Autodesk Inventor part; units mm, degrees
ref_plane "YZ Plane" through (0, 0, 0) normal (1, 0, 0) x (0, 1, 0)
ref_plane "XZ Plane" through (0, 0, 0) normal (0, 1, 0) x (-1, 0, 0)
ref_plane "XY Plane" through (0, 0, 0) normal (0, 0, 1) x (1, 0, 0)
sketch "Sketch1" plane through (0, 0, 0) normal (0, 0, 1) x (1, 0, 0)
  line L0 (-85, 15) -> (85, 15)
  line L1 (85, 15) -> (85, -15)
  line L2 (85, -15) -> (-85, -15)
  line L3 (-85, -15) -> (-85, 15)
  point P0 (0, 0)
  dimension "d0" = 30
  dimension "d1" = 170
  dimension "d2" = 85
  dimension "d3" = 15
extrude "Extrusion1" add sketch "Sketch1" along normal blind 10
sketch "Sketch2" plane through (0, 0, 10) normal (0, 0, 1) x (1, 0, 0)
  point P0 (0, 0)
  point P1 (-37.5, 0)
  point P2 (-12.5, 0)
  point P3 (12.5, 0)
  point P4 (37.5, 0)
  dimension "d30" = 25
  dimension "d31" = 25
  dimension "d32" = 25
  dimension "d33" = 12.5
hole "Hole1" at (-37.5, 0, 10) at (-12.5, 0, 10) at (12.5, 0, 10) at (37.5, 0, 10) direction (0, 0, -1) diameter 6.6 end through all counterbore diameter 18 counterbore depth 7
sketch "Sketch3" plane through (0, 0, 10) normal (0, 0, 1) x (1, 0, 0)
  point P0 (0, 0)
  point P1 (75, 0)
  point P2 (-75, 0)
  dimension "d16" = 150
  dimension "d17" = 75
hole "Hole2" at (75, 0, 10) at (-75, 0, 10) direction (0, 0, -1) diameter 3.242 end through all
properties part number "zStackJackAttach_Oct2016"
CAD build for the part. Positions are in the model's coordinates, mm. A direction names the side the tool comes from. Give positions to 0.01 mm unless a question says otherwise; leave off trailing zeros. Write each loop counter-clockwise with the first axis right and the second up, starting at its lowest first coordinate (ties: lowest second). Pieces come first, ordered by that corner, then holes. Notation, with made-up numbers: M 12,41 L 16,41 A10 cw 16,51 Z; hole C 39.5,80.5 d8. An arc over 180 degrees is marked long. Return JSON: item names as keys, results as strings. Group by question number.
(1) Band-saw the part on B-B (y = 0). State how many separate pieces and enclosed holes the cut face has, and give its area (3 significant figures).
(2) Band-saw the part on A-A (x = 12.5). Give the cut face in (y, z), and give its area (3 significant figures).
(3) Mould opens along X. For faces 1 (the face through (-46.423, 1.172, 6.451)), 2 (the face through (85, 0, 5)), 3 (the face through (-7.02, 7.14, 6.45)), 4 (the face through (-1, 0, 0)) say: pulls with the +X half, pulls with the -X half, needs draft (parallel to the pull), parting line crosses it, or undercut.
(4) Flat gauge pins, fed straight in: pin 1 Ø8.5 at (x, y) = (12.5, 0) entering from +Z; pin 2 Ø5.5 at (x, y) = (-37.5, 0) entering from -Z. Where does each tip first touch, or does it go through?
(5) Drill centre lines: L1, parallel to Y at x = -37.5, z = 1.6; L2, parallel to Y at x = 12.5, z = 6.75; L3, parallel to X at y = 7.5, z = 4. Where is each one in solid material? Low to high. Write a range as [from, to].
(6) Band-saw the part on D-D (x = 36). Give the cut face in (y, z).
(7) 3-axis set-ups, long thin cutter, end or side, ignore diameter. For faces 5 (the face through (-73.418, 0.351, 4.93)), 6 (the face through (16, 0, 3)): which of +Z, -Z, +X, -X, +Y, -Y reach the whole face in a straight line?
(8) Band-saw the part on C-C (x = 75). Give the cut face in (y, z), and give its area (3 significant figures).
Entries:
{
 "1": {"separate pieces": "7", "enclosed holes": "0", "area": "1,050 mm^2"},
 "2": {"outline": "M -15,0 L -3.3,0 L -3.3,3 L -9,3 L -9,10 L -15,10 Z; M 3.3,0 L 15,0 L 15,10 L 9,10 L 9,3 L 3.3,3 Z", "area": "154 mm^2"},
 "3": {"face 1": "undercut", "face 2": "pulls with the +X half", "face 3": "undercut", "face 4": "needs draft"},
 "4": {"pin 1": "stops at z = 3", "pin 2": "passes through"},
 "5": {"L1": "y = [-15, -3.3], [3.3, 15]", "L2": "y = [-15, -9], [9, 15]", "L3": "x = [-85, -42.47], [-32.53, -17.47], [-7.53, 7.53], [17.47, 32.53], [42.47, 85]"},
 "6": {"outline": "M -15,0 L -2.94,0 L -2.94,3 L -8.87,3 L -8.87,10 L -15,10 Z; M 2.94,0 L 15,0 L 15,10 L 8.87,10 L 8.87,3 L 2.94,3 Z"},
 "7": {"face 5": "+Z, -Z", "face 6": "+Z"},
 "8": {"outline": "M -15,0 L -1.62,0 L -1.62,10 L -15,10 Z; M 1.62,0 L 15,0 L 15,10 L 1.62,10 Z", "area": "268 mm^2"}
}
